Here's how the part is built. I have some questions about the finished solid (model axes, mm). Face numbers are marked on the shaded views. Give positions to 0.01 mm unless a question says otherwise; leave off trailing zeros. Loops run counter-clockwise (first coordinate to the right, second up) from the corner with the lowest first, then second, coordinate; pieces in that order, holes last. Notation, with made-up numbers: (37, 44) - (43, 44) arc R4 ccw to (43, 50) - close; hole circle Ø4 at (41.25, 63). An arc over 180 degrees is marked (long way). One line per item, written item: value. Start each with the question number.
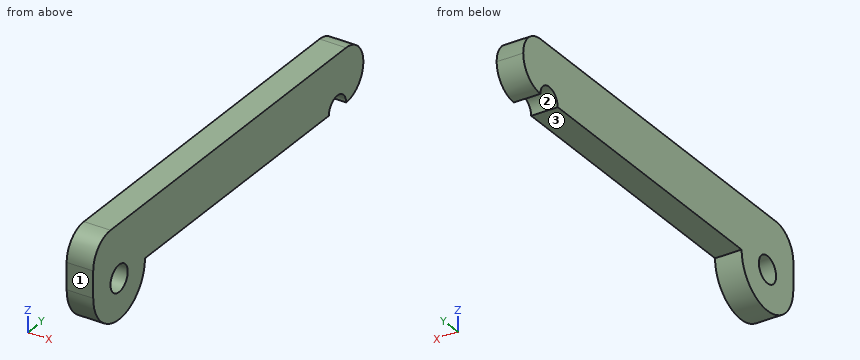
Autodesk Inventor part; units mm, degrees
ref_plane "YZ Plane" through (0, 0, 0) normal (1, 0, 0) x (0, 1, 0)
ref_plane "XZ Plane" through (0, 0, 0) normal (0, 1, 0) x (-1, 0, 0)
ref_plane "XY Plane" through (0, 0, 0) normal (0, 0, 1) x (1, 0, 0)
sketch "Sketch1" plane through (0, 0, 0) normal (1, 0, 0) x (0, 1, 0)
  line L0 (-4.5, 3) -> (4.5, 3)
  line L1 (4.5, 3) -> (4.5, -3)
  line L2 (4.5, -3) -> (-4.5, -3)
  line L3 (-4.5, -3) -> (-4.5, 3)
  line L4 (-4.5, 3) -> (4.5, -3) construction
  line L5 (4.5, 3) -> (-4.5, -3) construction
  circle A0 centre (0, -3) radius 4.5
  point P0 (0, 0)
  dimension "d0" = 9
  dimension "d1" = 6
  dimension "d2" = 9
extrude "Extrusion1" add sketch "Sketch1" along normal blind 3
sketch "Sketch2" plane through (3, 0, 0) normal (1, 0, 0) x (0, 0, -1)
  line L0 (3, 4.5) -> (-3, 4.5)
  line L1 (-3, 4.5) -> (-3, 42.5)
  line L2 (-3, 42.5) -> (3, 42.5)
  line L3 (3, 42.5) -> (3, 4.5)
  point P0 (0, 0)
  dimension "d5" = 6
  dimension "d6" = 38
extrude "Extrusion2" add sketch "Sketch2" against normal blind 3
sketch "Sketch3" plane through (3, 0, 0) normal (1, 0, 0) x (0, 0, -1)
  arc A0 (3, -4.5) -> (3, 4.5) centre (3, 0) ccw
  circle A1 centre (3, 0) radius 1.5
  point P0 (0, 0)
  dimension "d9" = 3
extrude "Extrusion3" cut sketch "Sketch3" against normal blind 3
fillet "Fillet1" radius 3 3 edges at (1.5, -4.5, 3) (1.5, 42.5, 3) (1.5, 42.5, -3)
sketch "Sketch4" plane through (0, 0, 0) normal (-1, 0, 0) x (0, 0, 1)
  circle A0 centre (-3, 38) radius 1.5
  circle A1 centre (-3, 0) radius 1.5
  point P0 (0, 0)
  dimension "d13" = 3
  dimension "d14" = 38
extrude "Extrusion4" cut sketch "Sketch4" against normal blind 3 contours A0
properties part number "Battery holder"
(1) Will these pins go through, and if not, where does the flat tip stop? pin 1 (1.5 mm diameter, centred on x = 1, z = -2, fed in from +Y); pin 2 (1.5 mm diameter, centred on x = 1, y = 19, fed in from -Z).
(2) If we mould it in two halves opening along Y, with no side actions, what happens to the marked faces 1, 2 and 3? For each: pulls with the +Y half, pulls with the -Y half, needs draft (parallel to the pull), parting line crosses it, or undercut.
(3) Please list where these lines run through material, in increasing order: probe 1 along Z at (x, y) = (0.75, 31.5); probe 2 along Y at (x, z) = (0.6, -2); probe 3 along Z at (x, y) = (0.5, 1). Write a range as from..to.
(4) If we section it at B-B on y = 7.5: List the corners of the cut face in (x, z) for me.
(5) If we section it at C-C on z = -6.25: List the corners of the cut face in (x, y) for me, plus the area to 3 significant figures.
Found:
1. pin 1: y = 42.23
1. pin 2: z = -3
2. face 1: pulls with the -Y half
2. face 2: undercut
2. face 3: needs draft
3. probe 1: -3..3
3. probe 2: -4.5..-1.12, 1.12..36.88, 39.12..41.74
3. probe 3: -7.39..-4.12, -1.88..3
4. outline: (0, -3) - (3, -3) - (3, 3) - (0, 3) - close
5. outline: (0, -3.11) - (3, -3.11) - (3, 3.11) - (0, 3.11) - close
5. area: 18.7 mm^2
